The model under review builds one solid part; all positions refer to its coordinate system, in mm. Round coordinates to 2 decimals unless told otherwise and drop trailing zeros. Write each loop counter-clockwise with the first axis right and the second up, starting at its lowest first coordinate (ties: lowest second). Pieces come first, ordered by that corner, then holes. Notation, with made-up numbers: (-15, 59) - (21, 59) arc R18 ccw to (21, 87) - close; hole circle Ø11 at (71, -13). An arc over 180 degrees is marked (long way). Write each question's results on one line, items separated by ' | '.
```python
from build123d import *

# Parameters (mm, degrees)
SKETCH2_R           = 5
SKETCH2_W           = 300
SKETCH2_H           = 300
BOSS_EXTRUDE1_DEPTH = 2


with BuildPart() as part:
    # Sketch2 → Boss-Extrude1 (new body)
    with BuildSketch(Plane.XY):
        with BuildLine():
            Line((-175, 190), (175, 190))
            ThreePointArc((175, 190), (185.606601718, 185.606601718), (190, 175))
            Line((190, 175), (190, -175))
            ThreePointArc((190, -175), (185.606601718, -185.606601718), (175, -190))
            Line((175, -190), (-175, -190))
            ThreePointArc((-175, -190), (-185.606601718, -185.606601718), (-190, -175))
            Line((-190, -175), (-190, 175))
            ThreePointArc((-190, 175), (-185.606601718, 185.606601718), (-175, 190))
        make_face()
        with Locations((-175, 175)):
            Circle(SKETCH2_R, mode=Mode.SUBTRACT)
        with Locations((0, 175)):
            Circle(SKETCH2_R, mode=Mode.SUBTRACT)
        with Locations((175, 175)):
            Circle(SKETCH2_R, mode=Mode.SUBTRACT)
        with Locations((175, 0)):
            Circle(SKETCH2_R, mode=Mode.SUBTRACT)
        with Locations((-175, 0)):
            Circle(SKETCH2_R, mode=Mode.SUBTRACT)
        with Locations((-175, -175)):
            Circle(SKETCH2_R, mode=Mode.SUBTRACT)
        with Locations((0, -175)):
            Circle(SKETCH2_R, mode=Mode.SUBTRACT)
        with Locations((175, -175)):
            Circle(SKETCH2_R, mode=Mode.SUBTRACT)
        Rectangle(SKETCH2_W, SKETCH2_H, mode=Mode.SUBTRACT)
    extrude(amount=BOSS_EXTRUDE1_DEPTH)


solid = part.part
```
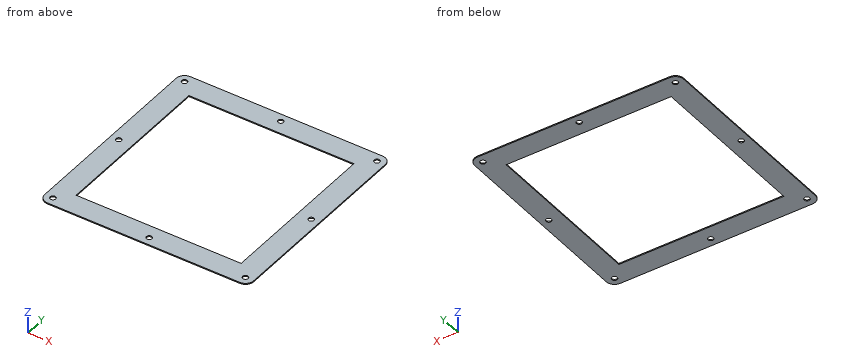
Q1. We need section D-D (z = 1.35). State how many separate pieces and enclosed holes the cut face has, plus the area to 3 significant figures.
Evaluation:
separate pieces: 1 | enclosed holes: 9 | area: 53,600 mm^2
Q2. For probe 1 along Y at (x, z) = (175, 1.15); probe 2 along Y at (x, z) = (0, 0.8); probe 3 along X at (y, z) = (-68, 0.75), list the stretches that pass through material, from the lowest coordinate up.
Evaluation:
probe 1: y = -190 to -180, -170 to -5, 5 to 170, 180 to 190 | probe 2: y = -190 to -180, -170 to -150, 150 to 170, 180 to 190 | probe 3: x = -190 to -150, 150 to 190
Q3. We need section A-A (x = 0). State the section outline as (y, z) points.
Evaluation:
outline: (-190, 0) - (-180, 0) - (-180, 2) - (-190, 2) - close; (-170, 0) - (-150, 0) - (-150, 2) - (-170, 2) - close; (150, 0) - (170, 0) - (170, 2) - (150, 2) - close; (180, 0) - (190, 0) - (190, 2) - (180, 2) - close
Q4. We need section C-C (y = 43.5). State the section outline as (x, z) points.
Evaluation:
outline: (-190, 0) - (-150, 0) - (-150, 2) - (-190, 2) - close; (150, 0) - (190, 0) - (190, 2) - (150, 2) - close
